Autodesk Inventor part; units mm, degrees
ref_plane "YZ Plane" through (0, 0, 0) normal (1, 0, 0) x (0, 1, 0)
ref_plane "XZ Plane" through (0, 0, 0) normal (0, 1, 0) x (-1, 0, 0)
ref_plane "XY Plane" through (0, 0, 0) normal (0, 0, 1) x (1, 0, 0)
sketch "Sketch1" plane through (0, 0, 0) normal (0, 0, 1) x (1, 0, 0)
  line L0 (48.2273, 127.3576) -> (98.2273, 127.3576)
  line L1 (98.2273, 127.3576) -> (98.2273, 105.3576)
  line L2 (98.2273, 105.3576) -> (48.2273, 105.3576)
  line L3 (48.2273, 105.3576) -> (48.2273, 127.3576)
  point P0 (0, 0)
  dimension "d8" = 50
  dimension "d9" = 22
extrude "Extrusion1" add sketch "Sketch1" along normal blind 5
sketch "Sketch2" plane through (98.2273, 105.3576, 0) normal (1, 0, 0) x (0, 0, -1)
  line L0 (-5, 0) -> (-50, 0)
  line L1 (-50, 0) -> (-50, 30)
  line L2 (-50, 30) -> (-20, 30)
  line L3 (-20, 30) -> (-20, 20)
  line L4 (-20, 20) -> (-45, 20)
  line L5 (-45, 20) -> (-45, 5)
  line L6 (-45, 5) -> (-5, 5)
  line L7 (-5, 0) -> (-5, 22)
  line L8 (-5, 5) -> (-5, 0)
  point P0 (0, -105.3576)
  dimension "d12" = 45
  dimension "d13" = 30
  dimension "d14" = 30
  dimension "d15" = 10
  dimension "d16" = 25
  dimension "d17" = 15
  dimension "d18" = 40
  dimension "d19" = 5
extrude "Extrusion2" add sketch "Sketch2" against normal blind 50
sketch "Sketch4" plane through (48.2273, 105.3576, 0) normal (0, -1, 0) x (1, 0, 0)
  line L0 (50, 50) -> (0, 50)
  circle A0 centre (25, 36) radius 2.65
  point P0 (-48.2273, 0)
  dimension "d24" = 5.3
extrude "Extrusion3" cut sketch "Sketch4" against normal blind 50
thread "Thread1"
thread "Thread2"
sketch "Sketch5" plane through (0, 0, 0) normal (0, 0, -1) x (-1, 0, 0)
  line L0 (-98.2273, 127.3576) -> (-48.2273, 127.3576)
  circle A0 centre (-73.2273, 120.7376) radius 3
  point P0 (0, 0)
  dimension "d32" = 6
extrude "Extrusion4" cut sketch "Sketch5" against normal blind 20
thread "Thread3"
properties part number "Chasis Depan Roda Kiri"
Read the model definition and answer for the solid it produces. Units are mm, in the model's axes. A direction names the side the tool comes from. Coordinates: 2 decimals unless noted, no trailing zeros. Loops run counter-clockwise (first coordinate to the right, second up) from the corner with the lowest first, then second, coordinate; pieces in that order, holes last.
Q1. The part is cut by section D-D on y = 129.75. Write down the section's boundary in (x, z), and give its area (3 significant figures).
Q2. Consider probe 1 along Y at (x, z) = (94, 33); probe 2 along Z at (x, y) = (73, 107); probe 3 along Z at (x, y) = (76, 115.5). Determine where each line is inside the solid, lowest interval first.
Q3. The part is cut by section A-A on y = 115.75. Write down the section's boundary in (x, z).
Q4. Each of these flat-tipped pins is pushed along its axis until it touches: pin 1 Ø8 at (y, z) = (123, 10) entering from +X; pin 2 Ø3 at (x, y) = (62, 129.5) entering from -Z; pin 3 Ø4 at (x, z) = (90.5, 8) entering from +Y; pin 4 Ø2.5 at (x, z) = (62.5, 1.5) entering from +Y. Where does it stop, or does it pass through?
Q5. Which of the six approach directions +Z, -Z, +X, -X, +Y, -Y give full straight-line access (tool end or side, diameter ignored) to faces 1 (the face through (73, 127.358, 2)), 2 (the face through (73, 117, 5)), 3 (the face through (75.755, 107.823, 36.796)), 4 (the face through (72, 118, 2)), 5 (the face through (74, 125.358, 32))?
Q6. The part is cut by section B-B on z = 36. Write down the section's boundary in (x, y).
Q7. The part is cut by section C-C on z = 27. Write down the section's boundary in (x, y).
Q8. The mould has two halves that part along Z. Classify faces 6 (the face through (74, 105.358, 25)), 7 (the face through (74, 120, 50)), 8 (the face through (74, 118, 45)): +Z half, -Z half, draft (parallel to the pull), parting line (faces both ways), or undercut.
Results below:
1. outline: (48.23, 20) - (98.23, 20) - (98.23, 50) - (48.23, 50) - close; hole circle Ø5.3 at (73.23, 36)
1. area: 1,480 mm2
2. probe 1: y = 105.36 to 110.36, 125.36 to 135.36
2. probe 2: z = 0 to 33.36, 38.64 to 50
2. probe 3: z = 0 to 5, 45 to 50
3. outline: (48.23, 0) - (98.23, 0) - (98.23, 5) - (48.23, 5) - close; (48.23, 45) - (98.23, 45) - (98.23, 50) - (48.23, 50) - close
4. pin 1: passes through
4. pin 2: stops at z = 20
4. pin 3: stops at y = 110.36
4. pin 4: stops at y = 127.36
5. face 1: -Z, +X, -X, +Y
5. face 2: +X, -X, +Y
5. face 3: +Y, -Y
5. face 4: -Z
5. face 5: +X, -X
6. outline: (48.23, 105.36) - (70.58, 105.36) - (70.58, 110.36) - (48.23, 110.36) - close; (48.23, 125.36) - (70.58, 125.36) - (70.58, 135.36) - (48.23, 135.36) - close; (75.88, 105.36) - (98.23, 105.36) - (98.23, 110.36) - (75.88, 110.36) - close; (75.88, 125.36) - (98.23, 125.36) - (98.23, 135.36) - (75.88, 135.36) - close
7. outline: (48.23, 105.36) - (98.23, 105.36) - (98.23, 110.36) - (48.23, 110.36) - close; (48.23, 125.36) - (98.23, 125.36) - (98.23, 135.36) - (48.23, 135.36) - close
8. face 6: draft
8. face 7: +Z half
8. face 8: undercut
